```python
from build123d import *

# Parameters (mm, degrees)
F3_DEPTH = 3
F4_R     = 3
F5_R     = 2


with BuildPart() as f3:
    # F0 (on Front) → F3 (new body, symmetric)
    with BuildSketch(Plane.XZ):
        with BuildLine():
            Line((0, -400), (0, 0))
            Line((0, 0), (-50, 0))
            Line((-50, 0), (-50, -400))
            Line((-50, -400), (-42.125, -400))
            Line((-42.125, -400), (-42.125, -405.6698729811))
            ThreePointArc((-42.125, -405.6698729811), (-39.625, -415), (-37.125, -405.6698729811))
            Line((-37.125, -405.6698729811), (-37.125, -400))
            Line((-37.125, -400), (-29.75, -400))
            Line((-29.75, -400), (-29.25, -385))
            Line((-29.25, -385), (-29.25, -30))
            Line((-29.25, -30), (-20.75, -30))
            Line((-20.75, -30), (-20.75, -385))
            Line((-20.75, -385), (-20.25, -400))
            Line((-20.25, -400), (-12.875, -400))
            Line((-12.875, -400), (-12.875, -394.3301270189))
            ThreePointArc((-12.875, -394.3301270189), (-10.375, -385), (-7.875, -394.3301270189))
            Line((-7.875, -394.3301270189), (-7.875, -400))
            Line((-7.875, -400), (0, -400))
        make_face()
    extrude(amount=F3_DEPTH, both=True)

    # F4
    f4_edges = [f3.edges().sort_by_distance(p)[0] for p in [
        (-50, 0, 0),
        (0, 0, 0),
        (-20.75, 0, -30),
        (-29.25, 0, -30),
    ]]
    fillet(f4_edges, radius=F4_R)

    # F5
    f5_edges = [f3.edges().sort_by_distance(p)[0] for p in [
        (-12.875, 0, -394.330127),
        (-12.875, 0, -400),
        (-37.125, 0, -400),
        (-7.875, 0, -400),
        (-7.875, 0, -394.330127),
        (-42.125, 0, -400),
        (-42.125, 0, -405.669873),
        (-37.125, 0, -405.669873),
    ]]
    fillet(f5_edges, radius=F5_R)


solid = f3.part
```
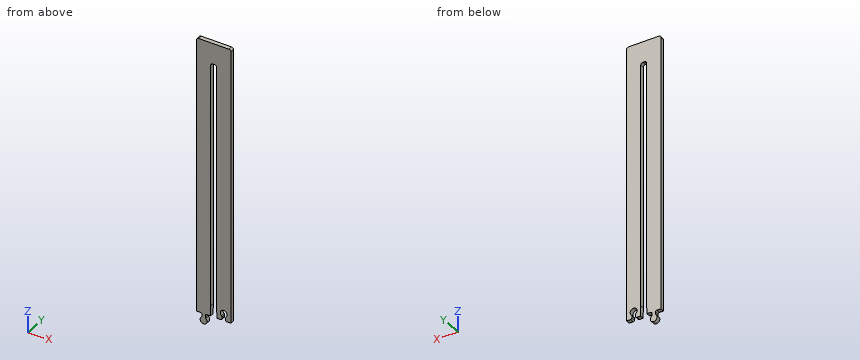
Work out the finished part from the listing and answer in its coordinate system (mm). Coordinates: 2 decimals unless noted, no trailing zeros. Write each loop counter-clockwise with the first axis right and the second up, starting at its lowest first coordinate (ties: lowest second). Pieces come first, ordered by that corner, then holes.
Q1. Find the intervals of material crossed by line 1 (X direction, y = 2.7, z = -186.5); line 2 (X direction, y = 1.3, z = -390) (3 decimals); line 3 (Z direction, x = -4, y = -1.45), in increasing order.
Q2. Each of these flat-tipped pins is pushed along its axis until it touches: pin 1 Ø0.8 at (y, z) = (0, -403) entering from +X (3 decimals); pin 2 Ø8 at (x, z) = (-10.375, -390) entering from -Y; pin 3 Ø1.3 at (y, z) = (1, -403) entering from -X (3 decimals); pin 4 Ø1.8 at (x, y) = (-3.5, 0.5) entering from -Z. Where does it stop, or does it pass through?
Q3. A cutting plane is placed at C-C, the plane z = -390. Give the vertices of the cut face in (x, y) (3 decimals), then the cut area to 3 significant figures.
Q4. A cutting plane is placed at A-A, the plane z = -280.5. Give the vertices of the cut face in (x, y), then the cut area to 3 significant figures.
Findings below:
1. line 1: x = -50 to -29.25, -20.75 to 0
1. line 2: x = -50 to -29.417, -20.583 to -15.375, -5.375 to 0
1. line 3: z = -400 to 0
2. pin 1: stops at x = -37.125
2. pin 2: passes through
2. pin 3: stops at x = -42.125
2. pin 4: stops at z = -400
3. outline: (-50, -3) - (-29.417, -3) - (-29.417, 3) - (-50, 3) - close; (-20.583, -3) - (-15.375, -3) - (-15.375, 3) - (-20.583, 3) - close; (-5.375, -3) - (0, -3) - (0, 3) - (-5.375, 3) - close
3. area: 187 mm2
4. outline: (-50, -3) - (-29.25, -3) - (-29.25, 3) - (-50, 3) - close; (-20.75, -3) - (0, -3) - (0, 3) - (-20.75, 3) - close
4. area: 249 mm2
